from build123d import *

# Parameters (mm, degrees)
F0_W     = 25.4
F0_H     = 25.4
F1_DEPTH = 25.4
F5_DEPTH = 25.401
F6_DEPTH = 25.401


with BuildPart() as f1:
    # F0 (on Top) → F1 (new body)
    with BuildSketch(Plane.XY):
        Rectangle(F0_W, F0_H)
    extrude(amount=F1_DEPTH)

    # F3 (on face) → F5 (intersect, through all)
    with BuildSketch(Plane(origin=(-12.7, 0, 0), x_dir=(0, -1, 0), z_dir=(-1, 0, 0))):
        Polygon((3.142383, 25.4), (0, 25.4), (-3.142383, 25.4), (-12.7, 0), (-7.581967, 0), (-5.010512, 6.833812), (0, 6.833812), (5.010512, 6.833812), (7.581967, 0), (12.7, 0), align=None)
        Polygon((-3.307431, 11.359861), (0, 20.149579), (3.307431, 11.359861), (0, 11.359861), align=None, mode=Mode.SUBTRACT)
    extrude(amount=-F5_DEPTH, mode=Mode.INTERSECT)

    # F4 (on face) → F6 (intersect, through all)
    with BuildSketch(Plane.XZ.offset(12.7)):
        with BuildLine():
            Line((-7.112893, 25.4), (-12.7, 25.4))
            Line((-12.7, 25.4), (-12.7, 0))
            Line((-12.7, 0), (-7.112893, 0))
            Line((-7.112893, 0), (-7.112893, 8.737554))
            Line((-7.112893, 8.737554), (2.215559, 8.737554))
            ThreePointArc((2.215559, 8.737554), (-2.51092, 10.208043), (-5.56892, 14.100417))
            Line((-5.56892, 14.100417), (-7.112893, 14.100417))
            Line((-7.112893, 14.100417), (-7.112893, 20.037137))
            Line((-7.112893, 20.037137), (-5.56892, 20.037137))
            ThreePointArc((-5.56892, 20.037137), (-2.51092, 23.929511), (2.215559, 25.4))
            Line((2.215559, 25.4), (-7.112893, 25.4))
        make_face()
        with BuildLine():
            ThreePointArc((10.546782, 17.068777), (8.106623, 22.959841), (2.215559, 25.4))
            ThreePointArc((2.215559, 25.4), (-2.51092, 23.929511), (-5.56892, 20.037137))
            Line((-5.56892, 20.037137), (2.299962, 20.037137))
            ThreePointArc((2.299962, 20.037137), (4.398909, 19.167725), (5.268321, 17.068777))
            ThreePointArc((5.268321, 17.068777), (4.398909, 14.96983), (2.299962, 14.100417))
            Line((2.299962, 14.100417), (-5.56892, 14.100417))
            ThreePointArc((-5.56892, 14.100417), (-2.51092, 10.208043), (2.215559, 8.737554))
            ThreePointArc((2.215559, 8.737554), (8.106623, 11.177713), (10.546782, 17.068777))
        make_face()
    extrude(amount=-F6_DEPTH, mode=Mode.INTERSECT)


solid = f1.part
Could you check a few things on this model? Use its own coordinates, in mm. A direction names the side the tool comes from. Give positions to 0.01 mm unless a question says otherwise; leave off trailing zeros. Write each loop counter-clockwise with the first axis right and the second up, starting at its lowest first coordinate (ties: lowest second). Pieces come first, ordered by that corner, then holes. Notation, with made-up numbers: (24, 50.5) -> (58, 50.5) arc R10 cw to (58, 61.5) -> close; hole circle Ø6 at (-31, 14). An arc over 180 degrees is marked (long way). Answer as CSV lines item,"result". Start each with the question number.
(1) Which directions (+Z, -Z, +X, -X, +Y, -Y) give clear straight access to the entire face, cutting with the end or side of a thin tool? Please do faces 4 (the face through (-2, 3, 20.037)), 5 (the face through (-3, 0, 8.738)), 6 (the face through (-2, 0, 11.36)), 7 (the face through (-9.95, -6.28, 3.46)).
(2) If we section it at C-C, the plane z = 3.5: Write out the boundary of the cut face in (x, y).
(3) If we section it at D-D, the plane y = -1.75: Write out the boundary of the cut face in (x, z), and give its area (3 significant figures).
(4) If we section it at A-A, the plane x = -3.5: Write out the boundary of the cut face in (y, z).
(5) Please list where these lines run through material, in increasing order: line 1 (Y direction, x = -7.25, z = 11.75); line 2 (Z direction, x = -6.75, y = 2); line 3 (X direction, y = 2, z = 7).
(6) If we mould it in two halves opening along Y, with no side actions, what happens to faces 1 (the face through (-2, -5, 14.1)), 2 (the face through (-1.24, 2.41, 13.74)), 3 (the face through (-3.822, 7.854, 12.878))? For each: +Y half, -Y half, draft (parallel to the pull), parting line (faces both ways), or undercut.
(7) If we section it at B-B, the plane x = -10.5: Write out the boundary of the cut face in (y, z), and give its area (3 significant figures).
(8) I'm going to push flat-ended pins straight in: pin 1 Ø3 at (x, y) = (-10, -1) entering from -Z; pin 2 Ø8 at (x, z) = (-1.5, 19) entering from -Y; pin 3 Ø4.5 at (x, y) = (-4.5, 1.5) entering from -Z. Where does each tip first touch, or does it pass through?
Answer list:
1,face 4,"+Y, -Y"
1,face 5,"-Z, +X, +Y, -Y"
1,face 6,"+X, -X"
1,face 7,"-Z, +X, -X"
2,outline,"(-12.7, -11.38) -> (-7.11, -11.38) -> (-7.11, -6.26) -> (-12.7, -6.26) -> close; (-12.7, 6.26) -> (-7.11, 6.26) -> (-7.11, 11.38) -> (-12.7, 11.38) -> close"
3,outline,"(-12.7, 6.83) -> (-7.11, 6.83) -> (-7.11, 8.74) -> (2.22, 8.74) arc R8.33 ccw to (8.28, 11.36) -> (-12.7, 11.36) -> close; (-12.7, 15.5) -> (-7.11, 15.5) -> (-7.11, 20.04) -> (2.3, 20.04) arc R2.97 cw to (5.27, 17.07) arc R2.97 cw to (4.82, 15.5) -> (10.4, 15.5) arc R8.33 ccw to (10.55, 17.07) arc R8.33 ccw to (2.22, 25.4) -> (-12.7, 25.4) -> close"
3,area,"222 mm^2"
4,outline,"(-9.41, 8.74) -> (9.41, 8.74) -> (7.39, 14.1) -> (2.28, 14.1) -> (3.31, 11.36) -> (-3.31, 11.36) -> (-2.28, 14.1) -> (-7.39, 14.1) -> close; (-5.16, 20.04) -> (-0.04, 20.04) -> (0, 20.15) -> (0.04, 20.04) -> (5.16, 20.04) -> (3.14, 25.4) -> (-3.14, 25.4) -> close"
5,line 1,"-8.28 to -3.16, 3.16 to 8.28"
5,line 2,"8.74 to 11.36, 20.04 to 25.4"
5,line 3,"-12.7 to -7.11"
6,face 1,"draft"
6,face 2,"undercut"
6,face 3,"+Y half"
7,outline,"(-12.7, 0) -> (-7.58, 0) -> (-5.01, 6.83) -> (5.01, 6.83) -> (7.58, 0) -> (12.7, 0) -> (3.14, 25.4) -> (-3.14, 25.4) -> close; hole (-3.31, 11.36) -> (3.31, 11.36) -> (0, 20.15) -> close"
7,area,"287 mm^2"
8,pin 1,"z = 6.83"
8,pin 2,"y = -5.16"
8,pin 3,"z = 8.74"
